Check sheet for the modelled part. Datum: model origin and axes. Units: mm. A direction names the side the tool comes from. Give positions to 0.01 mm unless a question says otherwise; leave off trailing zeros. Loops run counter-clockwise (first coordinate to the right, second up) from the corner with the lowest first, then second, coordinate; pieces in that order, holes last. Notation, with made-up numbers: (84.5, 7) - (90.5, 7) arc R24 cw to (90.5, 41) - close; hole circle Ø8 at (-0.5, 24). An arc over 180 degrees is marked (long way). Answer in a Markdown table with one row per item. Add a question column.
(1) Go/stop test with flat-tipped pins: P1, Ø1, axis at x = -2.5, y = 5.5, coming from the +Z side; P2, Ø1.5, axis at y = 1.5, z = 6, coming from the -X side; P3, Ø4, axis at x = 17.5, z = 1.5, coming from the +Y side. Record where each tip stops, or that it passes through.
(2) Sectioned sample at D-D on x = 0. Enter the section's corners in (y, z).
(3) Draft check along X on faces 3 (the face through (0, 0, 0)), 4 (the face through (15.369, 0.986, 5.816)), 5 (the face through (16.107, 0.986, -0.183)), 6 (the face through (-2.44, 5.01, -0.54)). Enter one of: released by +X, released by -X, zero draft, split by the parting line, or undercut.
(4) Set-up check for faces 1 (the face through (0, 4, 0)), 2 (the face through (0, 6, 3)): record each of +Z, -Z, +X, -X, +Y, -Y from which the full face is reachable in a straight line by a thin tool's end or side.
(5) Sectioned sample at A-A on y = 0.9. Enter the section's corners in (x, z), then the cut area to 3 significant figures.
(6) Thickness scan on L1, parallel to X at y = 1.45, z = 0; L2, parallel to X at y = 5.05, z = 0; L3, parallel to X at y = 4.75, z = 2. Record the ranges inside material, lowest first.
(7) Sectioned sample at C-C on x = 17.5. Enter the section's corners in (y, z), then the cut area to 3 significant figures.
(8) Sectioned sample at B-B on z = 0. Enter the section's corners in (x, y).
from build123d import *

# Parameters (mm, degrees)
SKETCH_1_R          = 15
EXTRUDE_1_DEPTH     = 6
SKETCH_2_R          = 2.5
CUT_EXTRUDE_1_DEPTH = 2
SKETCH_3_R          = 1.40543951
EXTRUDE_2_DEPTH     = 2


with BuildPart() as part:
    # 草图1 → 凸台-拉伸1 (new body)
    with BuildSketch(Plane(origin=(0, 0, 0), x_dir=(1, 0, 0), z_dir=(0, 1, 0))):
        with Locations(Location((0, 0, 0), (0, 0, 270))):
            Circle(SKETCH_1_R)
    extrude(amount=EXTRUDE_1_DEPTH)

    # 草图2 → 切除-拉伸1 (cut)
    with BuildSketch(Plane(origin=(0, 6, 0), x_dir=(1, 0, 0), z_dir=(0, 1, 0))):
        with Locations(Location((0, 0, 0), (0, 0, 270))):
            Circle(SKETCH_2_R)
    extrude(amount=-CUT_EXTRUDE_1_DEPTH, mode=Mode.SUBTRACT)

    # 草图3 → 凸台-拉伸2 (add)
    # profile 1 of 2: a face of its own
    with BuildSketch(Plane.XZ):
        with BuildLine():
            Line((-9.417192288, 11.675465276), (-19.104721401, 2.137790407))
            ThreePointArc((-19.104721401, 2.137790407), (-20, 0), (-19.104721401, -2.137790407))
            Line((-19.104721401, -2.137790407), (-9.417192288, -11.675465276))
            Line((-9.417192288, -11.675465276), (-9.417192288, 11.675465276))
        make_face()
        with Locations(Location((-17.5, 0, 0), (0, 0, 270))):
            Circle(SKETCH_3_R, mode=Mode.SUBTRACT)
    # profile 2 of 2: a face of its own
    with BuildSketch(Plane.XZ):
        with BuildLine():
            Line((9.417192288, 11.675465276), (9.417192288, -11.675465276))
            Line((9.417192288, -11.675465276), (19.104721401, -2.137790407))
            ThreePointArc((19.104721401, -2.137790407), (20, 0), (19.104721401, 2.137790407))
            Line((19.104721401, 2.137790407), (9.417192288, 11.675465276))
        make_face()
        with Locations(Location((17.5, 0, 0), (0, 0, 90))):
            Circle(SKETCH_3_R, mode=Mode.SUBTRACT)
    extrude(amount=-EXTRUDE_2_DEPTH)


solid = part.part
Reply:
| question | item | result |
|---|---|---|
| 1 | P1 | z = 14.87 |
| 1 | P2 | x = -15.94 |
| 1 | P3 | y = 2 |
| 2 | outline | (0, -15) - (6, -15) - (6, -2.5) - (4, -2.5) - (4, 2.5) - (6, 2.5) - (6, 15) - (0, 15) - close |
| 3 | face 3 | zero draft |
| 3 | face 4 | released by +X |
| 3 | face 5 | undercut |
| 3 | face 6 | undercut |
| 4 | face 1 | +Y |
| 4 | face 2 | +Z, -Z, +X, -X, +Y |
| 5 | outline | (-19.1, -2.14) - (-11.53, -9.6) arc R15 ccw to (11.53, -9.6) - (19.1, -2.14) arc R3 ccw to (19.1, 2.14) - (11.53, 9.6) arc R15 ccw to (-11.53, 9.6) - (-19.1, 2.14) arc R3 ccw to start; hole circle Ø2.81 at (-17.5, 0); hole circle Ø2.81 at (17.5, 0) |
| 5 | area | 786 mm^2 |
| 6 | L1 | -20 to -18.91, -16.09 to 16.09, 18.91 to 20 |
| 6 | L2 | -15 to -2.5, 2.5 to 15 |
| 6 | L3 | -14.87 to -1.5, 1.5 to 14.87 |
| 7 | outline | (0, -3.72) - (2, -3.72) - (2, -1.41) - (0, -1.41) - close; (0, 1.41) - (2, 1.41) - (2, 3.72) - (0, 3.72) - close |
| 7 | area | 9.25 mm^2 |
| 8 | outline | (-20, 0) - (-18.91, 0) - (-18.91, 2) - (-20, 2) - close; (-16.09, 0) - (16.09, 0) - (16.09, 2) - (15, 2) - (15, 6) - (2.5, 6) - (2.5, 4) - (-2.5, 4) - (-2.5, 6) - (-15, 6) - (-15, 2) - (-16.09, 2) - close; (18.91, 0) - (20, 0) - (20, 2) - (18.91, 2) - close |
